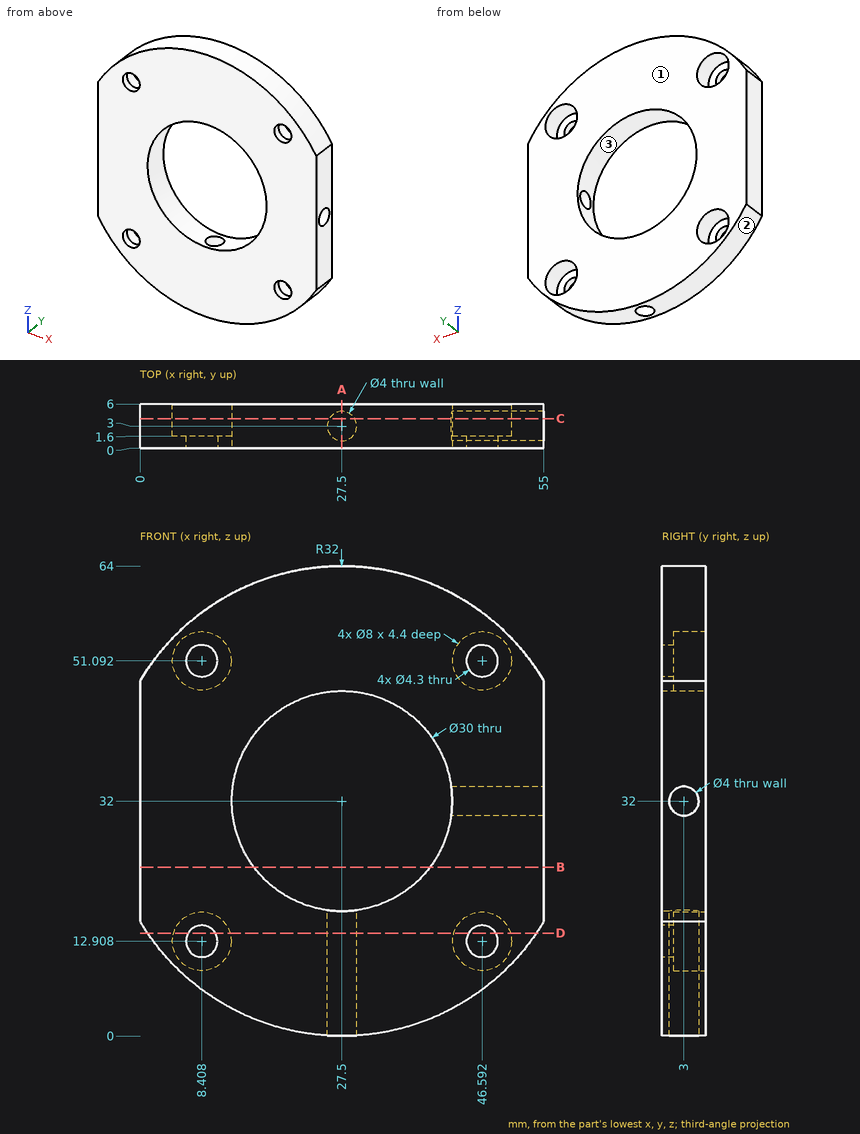
Print and shaded views of the part. All mm, measured from the part's lowest x, y and z. Coordinates: 2 decimals unless noted, no trailing zeros. Loops run counter-clockwise (first coordinate to the right, second up) from the corner with the lowest first, then second, coordinate; pieces in that order, holes last. Notation, with made-up numbers: (3, -13.5) - (11, -13.5) arc R22 ccw to (11, 14.5) - close; hole circle Ø4 at (56, 58). An arc over 180 degrees is marked (long way). Write item = value, one per line. Start each with the question number.
Item 1: Cut at C-C, the plane y = 4. Give the cut face in (x, z).
Item 2: Mould opens along X. For the marked faces 1, 2 and 3 say: released by +X, released by -X, zero draft, split by the parting line, or undercut.
Item 3: Wall check: L1, parallel to X at y = 1.75, z = 16; L2, parallel to X at y = 5.75, z = 32.5; L3, parallel to Y at x = 45, z = 32. Give the ranges that are in metal, low to high. Write a range as from..to.
Item 4: Cut at B-B, the plane z = 23. Give the cut face in (x, y), and give its area (3 significant figures).
Item 5: Cut at A-A, the plane x = 27.5. Give the cut face in (y, z).
Item 6: Cut at D-D, the plane z = 14. Give the cut face in (x, y), and give its area (3 significant figures).
Item 7: Flat gauge pins, fed straight in: pin 1 Ø4 at (x, z) = (7, 13) entering from +Y; pin 2 Ø3 at (y, z) = (3, 32) entering from +X; pin 3 Ø3.5 at (x, z) = (46.59, 12.91) entering from -Y; pin 4 Ø1 at (x, y) = (17.5, 1.5) entering from -Z. Where does each tip first touch, or does it go through?
The answers:
q1.outline = (0, 15.64) arc R32 ccw to (25.77, 0.05) - (25.77, 17.1) arc R15 cw (long way) to (42.4, 33.73) - (55, 33.73) - (55, 48.36) arc R32 ccw to (0, 48.36) - close; (29.23, 0.05) arc R32 ccw to (55, 15.64) - (55, 30.27) - (42.4, 30.27) arc R15 cw to (29.23, 17.1) - close; hole circle Ø8 at (8.41, 12.91); hole circle Ø8 at (8.41, 51.09); hole circle Ø8 at (46.59, 12.91); hole circle Ø8 at (46.59, 51.09)
q2.face_1 = zero draft
q2.face_2 = split by the parting line
q2.face_3 = undercut
q3.L1 = 0..5.87, 10.95..25.94, 29.06..44.05, 49.13..55
q3.L2 = 0..12.51, 42.49..55
q3.L3 = 0..1, 5..6
q4.outline = (0, 0) - (15.5, 0) - (15.5, 6) - (0, 6) - close; (39.5, 0) - (55, 0) - (55, 6) - (39.5, 6) - close
q4.area = 186 mm2
q5.outline = (0, 0) - (1, 0) - (1, 17) - (0, 17) - close; (0, 47) - (6, 47) - (6, 64) - (0, 64) - close; (5, 0) - (6, 0) - (6, 17) - (5, 17) - close
q6.outline = (1.04, 0) - (6.56, 0) - (6.56, 1.6) - (4.56, 1.6) - (4.56, 6) - (1.04, 6) - close; (10.26, 0) - (44.74, 0) - (44.74, 1.6) - (42.74, 1.6) - (42.74, 6) - (12.26, 6) - (12.26, 1.6) - (10.26, 1.6) - close; (48.44, 0) - (53.96, 0) - (53.96, 6) - (50.44, 6) - (50.44, 1.6) - (48.44, 1.6) - close; hole circle Ø4 at (27.5, 3)
q6.area = 225 mm2
q7.pin_1 = 1.6
q7.pin_2 = 12.58
q7.pin_3 = through
q7.pin_4 = 1.44
